```python
from build123d import *

# Parameters (mm, degrees)
BOSS_EXTRUDE1_DEPTH     = 13
BOSS_EXTRUDE1_2_DEPTH   = 13
BOSS_EXTRUDE2_DEPTH     = 1
CUT_EXTRUDE1_DEPTH      = 1
CUT_EXTRUDE1_DEPTH_BACK = 15
SKETCH5_R               = 2.95
CUT_EXTRUDE2_DEPTH      = 4
SKETCH6_R               = 1.7
CUT_EXTRUDE3_DEPTH      = 15
SKETCH7_R               = 2.95
CUT_EXTRUDE4_DEPTH      = 5
FILLET1_R               = 0.7


with BuildPart() as part:
    # Sketch1 → Boss-Extrude1 (new body)
    with BuildSketch(Plane.XY):
        with BuildLine():
            Line((20.312335657, 66.943000793), (-0.059999997, 66.943000793))
            ThreePointArc((-0.059999997, 66.943000793), (-2.501129835, 66.102927517), (-4.873699875, 65.085209777))
            Line((-4.873699875, 65.085209777), (-4.873699875, 59.450000396))
            Line((-4.873699875, 59.450000396), (25.126300125, 59.450000396))
            Line((25.126300125, 59.450000396), (25.126300125, 65.073261004))
            ThreePointArc((25.126300125, 65.073261004), (22.753848848, 66.097036745), (20.312335657, 66.943000793))
        make_face()
    extrude(amount=BOSS_EXTRUDE1_DEPTH)



with BuildPart() as body_2:
    # Sketch1 → Boss-Extrude1 2 (new body)
    with BuildSketch(Plane.XY):
        with BuildLine():
            Line((-4.873699875, 7.450000396), (25.126300125, 7.450000396))
            Line((25.126300125, 7.450000396), (25.126300125, 1.826739788))
            ThreePointArc((25.126300125, 1.826739788), (22.753848848, 0.802964047), (20.312335657, -0.043000001))
            Line((20.312335657, -0.043000001), (-0.059999997, -0.043000001))
            ThreePointArc((-0.059999997, -0.043000001), (-2.501129835, 0.797073275), (-4.873699875, 1.814791015))
            Line((-4.873699875, 1.814791015), (-4.873699875, 7.450000396))
        make_face()
    extrude(amount=BOSS_EXTRUDE1_2_DEPTH)


with BuildPart() as part_1:
    add(part.part)

    add(body_2.part)  # Boss-Extrude2 merges body 2
    # Sketch2 → Boss-Extrude2 (add)
    with BuildSketch(Plane.XY.offset(13)):
        with BuildLine():
            Line((-4.873699875, 7.450000396), (-4.873699875, 1.814791015))
            ThreePointArc((-4.873699875, 1.814791015), (-2.501129835, 0.797073275), (-0.059999997, -0.043000001))
            Line((-0.059999997, -0.043000001), (20.312335657, -0.043000001))
            ThreePointArc((20.312335657, -0.043000001), (22.753848848, 0.802964047), (25.126300125, 1.826739788))
            Line((25.126300125, 1.826739788), (25.126300125, 7.450000396))
            Line((25.126300125, 7.450000396), (25.126300125, 59.450000396))
            Line((25.126300125, 59.450000396), (25.126300125, 65.073261004))
            ThreePointArc((25.126300125, 65.073261004), (22.753848848, 66.097036745), (20.312335657, 66.943000793))
            Line((20.312335657, 66.943000793), (-0.059999997, 66.943000793))
            ThreePointArc((-0.059999997, 66.943000793), (-2.501129835, 66.102927517), (-4.873699875, 65.085209777))
            Line((-4.873699875, 65.085209777), (-4.873699875, 59.450000396))
            Line((-4.873699875, 59.450000396), (-4.873699875, 7.450000396))
        make_face()
    boss_extrude2 = extrude(amount=BOSS_EXTRUDE2_DEPTH)

    # Mirror1: Boss-Extrude2 across plane
    add(boss_extrude2.mirror(Plane(origin=(0, 0, 6.5), x_dir=(1, 0, 0), z_dir=(0, 0, -1))))

    # Sketch3 → Cut-Extrude1 (cut, two sides)
    with BuildSketch(Plane.XY.offset(14)) as cut_extrude1_sk:
        with BuildLine():
            Line((19.426300125, 40.450000396), (0.826300125, 40.450000396))
            ThreePointArc((0.826300125, 40.450000396), (0.331325379, 40.655025649), (0.126300125, 41.150000396))
            Line((0.126300125, 41.150000396), (0.126300125, 41.750000396))
            ThreePointArc((0.126300125, 41.750000396), (0.331325379, 42.244975143), (0.826300125, 42.450000396))
            Line((0.826300125, 42.450000396), (19.426300125, 42.450000396))
            ThreePointArc((19.426300125, 42.450000396), (19.921274872, 42.244975143), (20.126300125, 41.750000396))
            Line((20.126300125, 41.750000396), (20.126300125, 41.150000396))
            ThreePointArc((20.126300125, 41.150000396), (19.921274872, 40.655025649), (19.426300125, 40.450000396))
        make_face()
        with BuildLine():
            Line((19.426300125, 32.450000396), (0.826300125, 32.450000396))
            ThreePointArc((0.826300125, 32.450000396), (0.331325379, 32.655025649), (0.126300125, 33.150000396))
            Line((0.126300125, 33.150000396), (0.126300125, 33.750000396))
            ThreePointArc((0.126300125, 33.750000396), (0.331325379, 34.244975143), (0.826300125, 34.450000396))
            Line((0.826300125, 34.450000396), (19.426300125, 34.450000396))
            ThreePointArc((19.426300125, 34.450000396), (19.921274872, 34.244975143), (20.126300125, 33.750000396))
            Line((20.126300125, 33.750000396), (20.126300125, 33.150000396))
            ThreePointArc((20.126300125, 33.150000396), (19.921274872, 32.655025649), (19.426300125, 32.450000396))
        make_face()
        with BuildLine():
            Line((19.426300125, 48.450000396), (0.826300125, 48.450000396))
            ThreePointArc((0.826300125, 48.450000396), (0.331325379, 48.655025649), (0.126300125, 49.150000396))
            Line((0.126300125, 49.150000396), (0.126300125, 49.750000396))
            ThreePointArc((0.126300125, 49.750000396), (0.331325379, 50.244975143), (0.826300125, 50.450000396))
            Line((0.826300125, 50.450000396), (19.426300125, 50.450000396))
            ThreePointArc((19.426300125, 50.450000396), (19.921274872, 50.244975143), (20.126300125, 49.750000396))
            Line((20.126300125, 49.750000396), (20.126300125, 49.150000396))
            ThreePointArc((20.126300125, 49.150000396), (19.921274872, 48.655025649), (19.426300125, 48.450000396))
        make_face()
        with BuildLine():
            Line((19.426300125, 56.450000396), (0.826300125, 56.450000396))
            ThreePointArc((0.826300125, 56.450000396), (0.331325379, 56.655025649), (0.126300125, 57.150000396))
            Line((0.126300125, 57.150000396), (0.126300125, 57.750000396))
            ThreePointArc((0.126300125, 57.750000396), (0.331325379, 58.244975143), (0.826300125, 58.450000396))
            Line((0.826300125, 58.450000396), (19.426300125, 58.450000396))
            ThreePointArc((19.426300125, 58.450000396), (19.921274872, 58.244975143), (20.126300125, 57.750000396))
            Line((20.126300125, 57.750000396), (20.126300125, 57.150000396))
            ThreePointArc((20.126300125, 57.150000396), (19.921274872, 56.655025649), (19.426300125, 56.450000396))
        make_face()
        with BuildLine():
            Line((19.426300125, 24.450000396), (0.826300125, 24.450000396))
            ThreePointArc((0.826300125, 24.450000396), (0.331325379, 24.655025649), (0.126300125, 25.150000396))
            Line((0.126300125, 25.150000396), (0.126300125, 25.750000396))
            ThreePointArc((0.126300125, 25.750000396), (0.331325379, 26.244975143), (0.826300125, 26.450000396))
            Line((0.826300125, 26.450000396), (19.426300125, 26.450000396))
            ThreePointArc((19.426300125, 26.450000396), (19.921274872, 26.244975143), (20.126300125, 25.750000396))
            Line((20.126300125, 25.750000396), (20.126300125, 25.150000396))
            ThreePointArc((20.126300125, 25.150000396), (19.921274872, 24.655025649), (19.426300125, 24.450000396))
        make_face()
        with BuildLine():
            Line((19.426300125, 16.450000396), (0.826300125, 16.450000396))
            ThreePointArc((0.826300125, 16.450000396), (0.331325379, 16.655025649), (0.126300125, 17.150000396))
            Line((0.126300125, 17.150000396), (0.126300125, 17.750000396))
            ThreePointArc((0.126300125, 17.750000396), (0.331325379, 18.244975143), (0.826300125, 18.450000396))
            Line((0.826300125, 18.450000396), (19.426300125, 18.450000396))
            ThreePointArc((19.426300125, 18.450000396), (19.921274872, 18.244975143), (20.126300125, 17.750000396))
            Line((20.126300125, 17.750000396), (20.126300125, 17.150000396))
            ThreePointArc((20.126300125, 17.150000396), (19.921274872, 16.655025649), (19.426300125, 16.450000396))
        make_face()
        with BuildLine():
            Line((19.426300125, 8.450000396), (0.826300125, 8.450000396))
            ThreePointArc((0.826300125, 8.450000396), (0.331325379, 8.655025649), (0.126300125, 9.150000396))
            Line((0.126300125, 9.150000396), (0.126300125, 9.750000396))
            ThreePointArc((0.126300125, 9.750000396), (0.331325379, 10.244975143), (0.826300125, 10.450000396))
            Line((0.826300125, 10.450000396), (19.426300125, 10.450000396))
            ThreePointArc((19.426300125, 10.450000396), (19.921274872, 10.244975143), (20.126300125, 9.750000396))
            Line((20.126300125, 9.750000396), (20.126300125, 9.150000396))
            ThreePointArc((20.126300125, 9.150000396), (19.921274872, 8.655025649), (19.426300125, 8.450000396))
        make_face()
    extrude(amount=CUT_EXTRUDE1_DEPTH, mode=Mode.SUBTRACT)
    extrude(cut_extrude1_sk.sketch, amount=-CUT_EXTRUDE1_DEPTH_BACK, mode=Mode.SUBTRACT)

    # Sketch5 → Cut-Extrude2 (cut)
    with BuildSketch(Plane.XY.offset(14)):
        with Locations((10.126233978, 3.703500197)):
            Circle(SKETCH5_R)
    cut_extrude2 = extrude(amount=-CUT_EXTRUDE2_DEPTH, mode=Mode.SUBTRACT)

    # Sketch6 → Cut-Extrude3 (cut)
    with BuildSketch(Plane(origin=(0, 0, -1), x_dir=(-1, 0, 0), z_dir=(0, 0, -1))):
        with Locations((-10.126233978, 3.703500197)):
            Circle(SKETCH6_R)
    cut_extrude3 = extrude(amount=-CUT_EXTRUDE3_DEPTH, mode=Mode.SUBTRACT)

    # Sketch7 → Cut-Extrude4 (cut)
    with BuildSketch(Plane(origin=(0, 0, -1), x_dir=(-1, 0, 0), z_dir=(0, 0, -1))):
        with Locations((-10.126233978, 3.703500197)):
            Circle(SKETCH7_R)
    cut_extrude4 = extrude(amount=-CUT_EXTRUDE4_DEPTH, mode=Mode.SUBTRACT)

    # Mirror3: Cut-Extrude2, Cut-Extrude3, Cut-Extrude4 across plane
    add(cut_extrude2.mirror(Plane(origin=(0, 33.450000396, 0), x_dir=(0, 0, 1), z_dir=(0, -1, 0))), mode=Mode.SUBTRACT)
    add(cut_extrude3.mirror(Plane(origin=(0, 33.450000396, 0), x_dir=(0, 0, 1), z_dir=(0, -1, 0))), mode=Mode.SUBTRACT)
    add(cut_extrude4.mirror(Plane(origin=(0, 33.450000396, 0), x_dir=(0, 0, 1), z_dir=(0, -1, 0))), mode=Mode.SUBTRACT)

    # Fillet1
    fillet1_edges = [part_1.edges().sort_by_distance(p)[0] for p in [
        (7.176233978, 3.703500197, 14),
        (13.076233978, 3.703500197, -1),
        (7.176233978, 63.196500595, 14),
        (13.076233978, 63.196500595, -1),
    ]]
    fillet(fillet1_edges, radius=FILLET1_R)


solid = part_1.part
```
Input: part model. Units: mm. Frame: model coordinates. A direction names the side the tool comes from. Round coordinates to 2 decimals unless told otherwise and drop trailing zeros. Loops run counter-clockwise (first coordinate to the right, second up) from the corner with the lowest first, then second, coordinate; pieces in that order, holes last.
1) Material intervals for line 1 (Y direction, x = 10, z = 12.5); line 2 (Y direction, x = 1.25, z = 1.75); line 3 (Z direction, x = 14.75, y = 39), sorted ascending.
Ans:
line 1: y = -0.04 to 0.76, 6.65 to 7.45, 59.45 to 60.25, 66.14 to 66.94
line 2: y = -0.04 to 7.45, 59.45 to 66.94
line 3: z = -1 to 0, 13 to 14
2) Pull-direction query (X, two-part tool) for faces 6 (the cylindrical face through (22.72, 0.79, 6.6)), 7 (the cylindrical face through (-2.467, 66.116, 6.605)), 8 (the flat face through (10.2, 65.1, 4)), 9 (the flat face through (10, 66.943, 7)); classes: released by +X, released by -X, zero draft, split by the parting line, or undercut.
Ans:
face 6: released by +X
face 7: released by -X
face 8: undercut
face 9: zero draft
3) Section query B-B on y = 22. Return the cut outline in (x, z).
Ans:
outline: (-4.87, -1) - (25.13, -1) - (25.13, 0) - (-4.87, 0) - close; (-4.87, 13) - (25.13, 13) - (25.13, 14) - (-4.87, 14) - close
4) Section query C-C on x = -0.75. Return the cut outline in (y, z), plus the area to 3 significant figures.
Ans:
outline: (0.17, -1) - (66.73, -1) - (66.73, 14) - (0.17, 14) - close; hole (7.45, 0) - (59.45, 0) - (59.45, 13) - (7.45, 13) - close
area: 322 mm2
5) Pin query (flat end, axial travel): pin 1 (1.8 mm diameter, centred on x = 9, y = 64, fed in from +Z). Return the tip coordinate at first contact, or that it passes through.
Ans:
pin 1: stops at z = 10
6) Section query D-D on x = 5.25. Count the separate pieces of the cut face and the enclosed holes in it, plus the area to 3 significant figures.
Ans:
separate pieces: 14
enclosed holes: 0
area: 301 mm2
7) Section query A-A on z = 7. Return the cut outline in (x, y), plus the area to 3 significant figures.
Ans:
outline: (-4.87, 1.81) arc R35 ccw to (-0.06, -0.04) - (20.31, -0.04) arc R35 ccw to (25.13, 1.83) - (25.13, 7.45) - (-4.87, 7.45) - close; (-4.87, 59.45) - (25.13, 59.45) - (25.13, 65.07) arc R35 ccw to (20.31, 66.94) - (-0.06, 66.94) arc R35 ccw to (-4.87, 65.09) - close; hole circle Ø3.4 at (10.13, 3.7); hole circle Ø3.4 at (10.13, 63.2)
area: 415 mm2
8) Set-up query: faces 1 (the flat face through (25.126, 33, 13.3)), 2 (the flat face through (10, -0.043, 7)), 3 (the flat face through (11, 2, 10)), 4 (the flat face through (9, 2, 4)), 5 (the flat face through (10, 28, 13)). Return all of +Z, -Z, +X, -X, +Y, -Y with unobstructed straight access to the full face (end or side cutting, diameter ignored); none if empty.
Ans:
face 1: +Z, -Z, +X, +Y, -Y
face 2: +Z, -Z, +X, -X, -Y
face 3: +Z
face 4: -Z
face 5: +X, -X
